Autodesk Inventor part; units mm, degrees
ref_plane "YZ Plane" through (0, 0, 0) normal (1, 0, 0) x (0, 1, 0)
ref_plane "XZ Plane" through (0, 0, 0) normal (0, 1, 0) x (-1, 0, 0)
ref_plane "XY Plane" through (0, 0, 0) normal (0, 0, 1) x (1, 0, 0)
sketch "Sketch1" plane through (0, 0, 0) normal (0, 0, 1) x (1, 0, 0)
  line L0 (0, 0) -> (38.1, 0)
  line L1 (38.1, 0) -> (38.1, -38.1)
  line L2 (38.1, -38.1) -> (0, -38.1)
  line L3 (0, -38.1) -> (0, 0)
  dimension "d0" = 38.1
  dimension "d1" = 38.1
extrude "Extrusion1" add sketch "Sketch1" along normal blind 1.6002
sketch "Sketch2" plane through (0, 0, 1.6002) normal (0, 0, 1) x (1, 0, 0)
  line L0 (38.1, 0) -> (0, 0)
  line L1 (0, 0) -> (0, -38.1)
  line L2 (0, -38.1) -> (38.1, -38.1)
  line L3 (38.1, -38.1) -> (38.1, 0)
  line L4 (9.525, -9.525) -> (28.575, -9.525)
  line L5 (28.575, -9.525) -> (28.575, -28.575)
  line L6 (28.575, -28.575) -> (9.525, -28.575)
  line L7 (9.525, -28.575) -> (9.525, -9.525)
  dimension "d4" = 9.525
  dimension "d5" = 9.525
  dimension "d6" = 9.525
  dimension "d7" = 9.525
extrude "Extrusion2" add sketch "Sketch2" along normal blind 7.62 contours L4 L5 L6 L7
sketch "Sketch3" plane through (0, 0, 9.2202) normal (0, 0, 1) x (1, 0, 0)
  circle A0 centre (19.05, -19.05) radius 6.985
  point P0 (0, 0)
  dimension "d10" = 13.97
extrude "Extrusion3" add sketch "Sketch3" along normal blind 20.32
properties part number "Camera" material "ABS Plastic"
Build history of the part. All positions in model axes, mm. A direction names the side the tool comes from. Round coordinates to 2 decimals unless told otherwise and drop trailing zeros. Write each loop counter-clockwise with the first axis right and the second up, starting at its lowest first coordinate (ties: lowest second). Pieces come first, ordered by that corner, then holes. Notation, with made-up numbers: (38.25, 29.5) -> (47.25, 29.5) arc R35 cw to (47.25, 68.5) -> close; hole circle Ø6 at (21.5, 64). An arc over 180 degrees is marked (long way). Use one line per item in the form item = value.
Q1. Band-saw the part on B-B, the plane y = -27. Write the cut outline in (x, z) (3 decimals), then the cut area to 3 significant figures.
Conclusion:
outline = (0, 0) -> (38.1, 0) -> (38.1, 1.6) -> (28.575, 1.6) -> (28.575, 9.22) -> (9.525, 9.22) -> (9.525, 1.6) -> (0, 1.6) -> close
area = 206 mm²
Q2. Drop flat-ended pins along their axis: P1, Ø4, axis at x = 20, z = 4, coming from the +Y side (3 decimals); P2, Ø2.5, axis at y = -17, z = 6, coming from the -X side (3 decimals); P3, Ø2, axis at y = -21.5, z = 10.5, coming from the +X side; P4, Ø8, axis at x = 8, y = -7, coming from the -Z side. Give the stop position or say it passes through.
Conclusion:
P1 = -9.525
P2 = 9.525
P3 = 25.88
P4 = 0
Q3. Band-saw the part on C-C, the plane z = 3.5. Write the cut outline in (x, y) (3 decimals).
Conclusion:
outline = (9.525, -28.575) -> (28.575, -28.575) -> (28.575, -9.525) -> (9.525, -9.525) -> close
Q4. Tool access for faces 1 (the flat face through (28.575, -19, 5)), 2 (the flat face through (19, -9.525, 5)), 3 (the flat face through (9.525, -19, 5)): list every direction of +Z, -Z, +X, -X, +Y, -Y with a clear straight run to the whole face (end or side of a thin tool).
Conclusion:
face_1 = +Z, +X, +Y, -Y
face_2 = +Z, +X, -X, +Y
face_3 = +Z, -X, +Y, -Y
Q5. Band-saw the part on A-A, the plane x = 19.05. Write the cut outline in (y, z) (3 decimals), then the cut area to 3 significant figures.
Conclusion:
outline = (-38.1, 0) -> (0, 0) -> (0, 1.6) -> (-9.525, 1.6) -> (-9.525, 9.22) -> (-12.065, 9.22) -> (-12.065, 29.54) -> (-26.035, 29.54) -> (-26.035, 9.22) -> (-28.575, 9.22) -> (-28.575, 1.6) -> (-38.1, 1.6) -> close
area = 490 mm²
Q6. Drill centre lines: L1, parallel to Z at x = 2, y = -12.5; L2, parallel to Z at x = 10, y = -27; L3, parallel to Y at x = 11, z = 7 (3 decimals). Where is each one in solid material? Low to high.
Conclusion:
L1 = 0 to 1.6
L2 = 0 to 9.22
L3 = -28.575 to -9.525
Q7. Band-saw the part on D-D, the plane x = 10.5. Write the cut outline in (y, z) (3 decimals), then the cut area to 3 significant figures.
Conclusion:
outline = (-38.1, 0) -> (0, 0) -> (0, 1.6) -> (-9.525, 1.6) -> (-9.525, 9.22) -> (-28.575, 9.22) -> (-28.575, 1.6) -> (-38.1, 1.6) -> close
area = 206 mm²
